Geometry check sheet. Reference: drawing and pictorial views, mm from the part's lowest x, y, z. A direction names the side the tool comes from. Give positions to 0.01 mm unless a question says otherwise; leave off trailing zeros. Order: outer loops, then holes, each group sorted by start corner. A loop starts at its lowest first (then second) coordinate and runs counter-clockwise, first axis right, second up. Notation, with made-up numbers: (49.5, 82.5) -> (85.5, 82.5) arc R33 ccw to (85.5, 116.5) -> close; hole circle Ø8 at (78, -29.75). An arc over 180 degrees is marked (long way). Write each question's results on one line, items separated by ' | '.
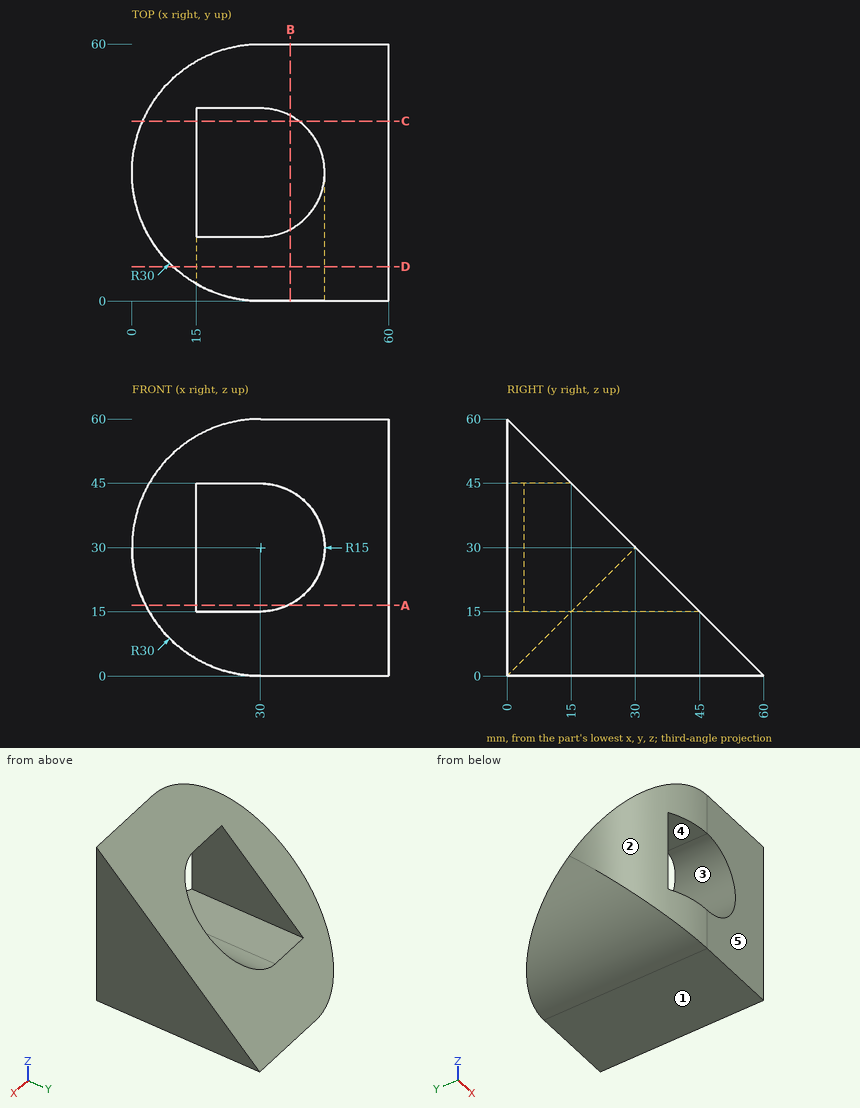
1. Access from +Z, -Z, +X, -X, +Y, -Y to the whole of each face (thin tool, end or side, straight path). Record for the marked faces 4 and 5.
Verdict:
face 4: +Y, -Y | face 5: +Z, -Z, +X, -X, -Y
2. Section check D-D on y = 8. Record the cut outline in (x, z), then the cut area to 3 significant figures.
Verdict:
outline: (9.6, 8) arc R30 ccw to (30, 0) -> (60, 0) -> (60, 52) -> (9.6, 52) -> close; hole (15, 15) -> (30, 15) arc R15 ccw to (30, 45) -> (15, 45) -> close | area: 1,770 mm^2
3. Section check A-A on z = 16.5. Record the cut outline in (x, y), then the cut area to 3 significant figures.
Verdict:
outline: (3.21, 16.5) arc R30 ccw to (15, 4.02) -> (15, 43.5) -> (3.21, 43.5) -> close; (36.54, 0) -> (60, 0) -> (60, 43.5) -> (36.54, 43.5) -> close | area: 1,430 mm^2
4. Section check C-C on y = 42. Record the cut outline in (x, z).
Verdict:
outline: (2.5, 18) arc R30 ccw to (30, 0) -> (60, 0) -> (60, 18) -> (39, 18) arc R15 cw to (30, 15) -> (15, 15) -> (15, 18) -> close
5. Gauge pin test, flat ends, axial feed: pin 1 Ø1.5 at (x, y) = (9, 42) entering from -Z; pin 2 Ø12 at (x, z) = (37, 33.5) entering from -Y; pin 3 Ø7.5 at (x, y) = (26, 20.5) entering from +Z; pin 4 Ø10 at (x, y) = (10, 31) entering from -Z. Record the tip position at first contact, or that the pin passes through.
Verdict:
pin 1: stops at z = 7.87 | pin 2: passes through | pin 3: stops at z = 15 | pin 4: stops at z = 4.02
6. Material ranges on probe 1 along Y at (x, z) = (38.5, 56); probe 2 along Y at (x, z) = (57.5, 15); probe 3 along X at (y, z) = (8, 38.5), recorded low to high. Write a range as from..to.
Verdict:
probe 1: y = 0..4 | probe 2: y = 0..45 | probe 3: x = 9.6..15, 42.36..60
7. Section check B-B on x = 37. Record the cut outline in (y, z), then the cut area to 3 significant figures.
Verdict:
outline: (0, 0) -> (60, 0) -> (43.27, 16.73) -> (0, 16.73) -> close; (0, 43.27) -> (16.73, 43.27) -> (0, 60) -> close | area: 1,000 mm^2
8. Mould release check, pull along X, two halves, no side actions. Record for the marked faces 1, 2 and 3: +X half, -X half, draft (parallel to the pull), parting line (faces both ways), or undercut.
Verdict:
face 1: draft | face 2: -X half | face 3: undercut
